Part model, mm, in its own coordinate system. Give positions to 0.01 mm unless a question says otherwise; leave off trailing zeros. Write each loop counter-clockwise with the first axis right and the second up, starting at its lowest first coordinate (ties: lowest second). Pieces come first, ordered by that corner, then holes. Notation, with made-up numbers: M 75.25,78.25 L 124.25,78.25 A31 ccw 124.25,115.25 Z; hole C 73,71 d11. An arc over 180 degrees is marked long. Use a Markdown table: item, result.
```python
from build123d import *

# Parameters (mm, degrees)
F0_W     = 228.6
F0_H     = 160.02
F1_DEPTH = 6.35
F2_R     = 61.9125
F3_DEPTH = 25.4
F4_R     = 3.175
F5_DEPTH = 25.4


with BuildPart() as f1:
    # F0 (on Top) → F1 (new body)
    with BuildSketch(Plane.XY):
        with Locations((0.783786, -1.108692)):
            Rectangle(F0_W, F0_H)
    extrude(amount=F1_DEPTH)

    # F2 (on face) → F3 (cut)
    with BuildSketch(Plane.XY.offset(6.35)):
        with Locations((27.771286, -1.108692)):
            Circle(F2_R)
    extrude(amount=-F3_DEPTH, mode=Mode.SUBTRACT)

    # F4 (on face) → F5 (cut)
    with BuildSketch(Plane.XY.offset(6.35)):
        with Locations((-88.116214, -23.333692)):
            Circle(F4_R)
        with Locations((-88.116214, -1.108692)):
            Circle(F4_R)
        with Locations((-88.116214, 21.116308)):
            Circle(F4_R)
    extrude(amount=-F5_DEPTH, mode=Mode.SUBTRACT)


solid = f1.part
```
1. Cut at A-A, the plane x = -9. Give the cut face in (y, z).
Findings below:
| item | result |
|---|---|
| outline | M -81.12,0 L -50.92,0 L -50.92,6.35 L -81.12,6.35 Z; M 48.7,0 L 78.9,0 L 78.9,6.35 L 48.7,6.35 Z |
2. Two-plate mould, pull along X, no slides. Class faces 1 (the flat face through (-113.516, -2, 3)), 2 (the flat face through (-1, 78.901, 3)), 3 (the cylindrical face through (-91.29, -0.97, 3.22)), 4 (the cylindrical face through (-91.288, 21.256, 3.219)): released by +X, released by -X, zero draft, split by the parting line, or undercut.
Findings below:
| item | result |
|---|---|
| face 1 | released by -X |
| face 2 | zero draft |
| face 3 | undercut |
| face 4 | undercut |
3. Drill centre lines: L1, parallel to Y at x = 25.5, z = 5.75; L2, parallel to Y at x = -0.5, z = 0.5; L3, parallel to X at y = 31.5, z = 1.25. Where is each one in solid material? Low to high.
Findings below:
| item | result |
|---|---|
| L1 | -81.12 to -62.98, 60.76 to 78.9 |
| L2 | -81.12 to -56.19, 53.97 to 78.9 |
| L3 | -113.52 to -24.86, 80.4 to 115.08 |
4. Cut at B-B, the plane y = -54. Give the cut face in (x, z).
Findings below:
| item | result |
|---|---|
| outline | M -113.52,0 L -4.41,0 L -4.41,6.35 L -113.52,6.35 Z; M 59.95,0 L 115.08,0 L 115.08,6.35 L 59.95,6.35 Z |
5. Cut at C-C, the plane z = 2. State how many separate pieces and enclosed holes the cut face has, then the cut area to 3 significant figures.
Findings below:
| item | result |
|---|---|
| separate pieces | 1 |
| enclosed holes | 4 |
| area | 24,400 mm2 |
